The listing builds one solid part. Answer for the finished solid, in the listing's coordinates (mm). Give positions to 0.01 mm unless a question says otherwise; leave off trailing zeros. Write each loop counter-clockwise with the first axis right and the second up, starting at its lowest first coordinate (ties: lowest second). Pieces come first, ordered by that corner, then holes. Notation, with made-up numbers: (-18, 21.5) -> (30, 21.5) arc R14 ccw to (30, 27.5) -> close; hole circle Ø3 at (-34, 84). An arc over 180 degrees is marked (long way). Put each result on its own line as item: value. Start each with the question number.
1) Find the intervals of material crossed by line 1 along X through (y, z) = (2, 1.1); line 2 along Y through (x, z) = (15, -0.6); line 3 along X through (y, z) = (8.5, 0.95), in increasing order. Write a range as from..to.
2) A cutting plane is placed at A-A (y = 15.5). Write down the section's boundary in (x, z), then the cut area to 3 significant figures.
3) A cutting plane is placed at C-C (x = -26.5). Write down the section's boundary in (y, z).
4) A cutting plane is placed at B-B (x = -45.5). Write down the section's boundary in (y, z).
5) Flat-ended cylindrical pins translate along their axes: pin 1 Ø0.9 at (y, z) = (6.5, -1) entering from +X; pin 2 Ø0.5 at (y, z) = (4.5, -0.5) entering from +X; pin 3 Ø3 at (x, y) = (-41.61, 16.5) entering from -Z; pin 4 Ø1.1 at (x, z) = (-32, 0.5) entering from -Y. Find the tip coordinate at first contact, or state that the pin passes through.
Autodesk Inventor part; units mm, degrees
sketch "Эскиз1" plane through (0, 0, 0) normal (0, 0, 1) x (1, 0, 0)
  line L0 (-70.2411, 0) -> (14.7589, 0)
  line L1 (14.7589, 0) -> (14.7589, 30)
  line L2 (14.7589, 30) -> (-70.2411, 20)
  line L3 (0, 36) -> (0, -6) construction
  line L4 (-70.2411, 20) -> (-70.2411, 0)
  point P0 (0, 0)
  dimension "d0" = 30
  dimension "d1" = 85
  dimension "d46" = 14.7589
  dimension "d47" = 20
extrude "Выдавливание1" add sketch "Эскиз1" along normal mid plane 4
sketch "Эскиз2" plane through (-70.2411, 0, 2) normal (0, -1, 0) x (1, 0, 0)
  line L0 (0, -4) -> (0, 0)
  line L1 (85, 0) -> (0, 0)
  line L2 (0, -4) -> (5, -4)
  line L3 (5, -4) -> (5, 0)
  line L4 (5, 0) -> (0, 0)
  line L5 (0, 0) -> (0, -4)
  line L6 (0, -4) -> (85, -4)
  line L7 (15, -4) -> (20, -4)
  line L8 (20, -4) -> (20, 0)
  line L9 (20, 0) -> (15, 0)
  line L10 (15, 0) -> (15, -4)
  line L11 (30, -4) -> (35, -4)
  line L12 (35, -4) -> (35, 0)
  line L13 (35, 0) -> (30, 0)
  line L14 (30, 0) -> (30, -4)
  line L15 (45, -4) -> (50, -4)
  line L16 (50, -4) -> (50, 0)
  line L17 (50, 0) -> (45, 0)
  line L18 (45, 0) -> (45, -4)
  line L19 (85, -4) -> (80, -4)
  line L20 (80, -4) -> (80, 0)
  line L21 (80, 0) -> (85, 0)
  line L22 (85, 0) -> (85, -4)
  line L23 (74, -4) -> (69, -4)
  line L24 (69, -4) -> (69, 0)
  line L25 (69, 0) -> (74, 0)
  line L26 (74, 0) -> (74, -4)
  point P0 (70.2411, -2)
  point P1 (15, 0)
  point P2 (45, 0)
  point P3 (74, 0)
  dimension "d4" = 5
  dimension "d5" = 5
  dimension "d6" = 10
  dimension "d9" = 30
  dimension "d14" = 5
  dimension "d15" = 5
  dimension "d16" = 6
extrude "Выдавливание2" add sketch "Эскиз2" along normal blind 3 contours L0 L1 L3 L2 | L10 L1 L8 L6 | L14 L1 L12 L6 | L18 L1 L16 L6 | L24 L1 L26 L6 | L20 L1 L22 L6
sketch "Эскиз3" plane through (14.7589, 30, 2) normal (1, 0, 0) x (0, 0, -1)
  line L0 (4, 0) -> (0, 0)
  line L1 (4, 0) -> (0, 0)
  line L2 (0, 0) -> (0, -4)
  line L3 (0, -4) -> (4, -4)
  line L4 (4, -4) -> (4, 0)
  line L5 (4, -9) -> (0, -9)
  line L6 (0, -9) -> (0, -13)
  line L7 (0, -13) -> (4, -13)
  line L8 (4, -13) -> (4, -9)
  line L9 (4, 0) -> (4, -33)
  line L10 (4, -10) -> (4, 0)
  line L11 (0, 0) -> (0, -33)
  line L12 (4, -17) -> (0, -17)
  line L13 (0, -17) -> (0, -21)
  line L14 (0, -21) -> (4, -21)
  line L15 (4, -21) -> (4, -17)
  line L16 (4, -26) -> (0, -26)
  line L17 (0, -26) -> (0, -30)
  line L18 (0, -30) -> (4, -30)
  line L19 (4, -30) -> (4, -26)
  point P0 (2, -30)
  point P1 (4, -30)
  point P2 (4, -16.5)
  point P3 (4, -30)
  point P4 (0, -26)
  point P5 (0, -17)
  dimension "d19" = 4
  dimension "d20" = 4
  dimension "d21" = 5
  dimension "d29" = 4
  dimension "d30" = 5
  dimension "d31" = 4
  dimension "d32" = 4
extrude "Выдавливание3" add sketch "Эскиз3" along normal blind 6 contours L4 L3 L2 L0 | L8 L7 L6 L5 | L12 L9 L14 L11 | L16 L9 L18 L11
sketch "Эскиз4" plane through (0, 0, 2) normal (0, 0, 1) x (1, 0, 0)
  line L0 (-0.1411, 5.05) -> (-0.1411, 7.95)
  line L1 (14.7589, 7.95) -> (14.7589, 5.05)
  line L2 (6.6589, 9.3) -> (4.8589, 9.3)
  line L3 (4.8589, 3.7) -> (6.6589, 3.7)
  line L4 (14.7589, 9) -> (14.7589, 4)
  line L5 (14.7589, 6.5) -> (-0.1411, 6.5) construction
  line L6 (-0.1411, 7.95) -> (4.8589, 7.95)
  line L7 (6.6589, 7.95) -> (14.7589, 7.95)
  line L8 (6.6589, 3.7) -> (6.6589, 5.05)
  line L9 (6.6589, 7.95) -> (6.6589, 9.3)
  line L10 (4.8589, 9.3) -> (4.8589, 7.95)
  line L11 (4.8589, 5.05) -> (4.8589, 3.7)
  line L12 (14.7589, 5.05) -> (6.6589, 5.05)
  line L13 (4.8589, 5.05) -> (-0.1411, 5.05)
  line L14 (-0.1411, 22.05) -> (-0.1411, 24.95)
  line L15 (14.7589, 24.95) -> (14.7589, 22.05)
  line L16 (6.6589, 26.3) -> (4.8589, 26.3)
  line L17 (4.8589, 20.7) -> (6.6589, 20.7)
  line L18 (14.7589, 23.5) -> (-0.1411, 23.5) construction
  line L19 (-0.1411, 24.95) -> (4.8589, 24.95)
  line L20 (6.6589, 24.95) -> (14.7589, 24.95)
  line L21 (6.6589, 20.7) -> (6.6589, 22.05)
  line L22 (6.6589, 24.95) -> (6.6589, 26.3)
  line L23 (4.8589, 26.3) -> (4.8589, 24.95)
  line L24 (4.8589, 22.05) -> (4.8589, 20.7)
  line L25 (14.7589, 22.05) -> (6.6589, 22.05)
  line L26 (4.8589, 22.05) -> (-0.1411, 22.05)
  line L27 (14.7589, 26) -> (14.7589, 21)
  point P0 (0, 0)
  dimension "d33" = 2.9
  dimension "d34" = 1.8
  dimension "d35" = 5.6
  dimension "d37" = 1.35
  dimension "d38" = 5
  dimension "d39" = 8.1
  dimension "d40" = 2.9
  dimension "d41" = 1.8
  dimension "d42" = 5.6
  dimension "d43" = 1.35
  dimension "d44" = 5
  dimension "d45" = 8.1
extrude "Выдавливание4" cut sketch "Эскиз4" against normal up to surface (4 mm away)
sketch "Эскиз5" plane through (0, 0, 2) normal (0, 0, 1) x (1, 0, 0)
  line L0 (-61.6911, 0) -> (-58.7911, 0)
  line L1 (-58.7911, 13.9) -> (-61.6911, 13.9)
  line L2 (-31.6911, 0) -> (-28.7911, 0)
  line L3 (-28.7911, 13.9) -> (-31.6911, 13.9)
  line L4 (-60.2411, 0) -> (-60.2411, 13.9) construction
  line L5 (-30.2411, 13.9) -> (-30.2411, 0) construction
  line L6 (-57.4411, 9.9) -> (-57.4411, 8.1)
  line L7 (-63.0411, 8.1) -> (-63.0411, 9.9)
  line L8 (-27.4411, 9.9) -> (-27.4411, 8.1)
  line L9 (-33.0411, 8.1) -> (-33.0411, 9.9)
  line L10 (-63.0411, 9.9) -> (-61.6911, 9.9)
  line L11 (-58.7911, 9.9) -> (-57.4411, 9.9)
  line L12 (-61.6911, 13.9) -> (-61.6911, 9.9)
  line L13 (-61.6911, 8.1) -> (-61.6911, 0)
  line L14 (-57.4411, 8.1) -> (-58.7911, 8.1)
  line L15 (-61.6911, 8.1) -> (-63.0411, 8.1)
  line L16 (-58.7911, 0) -> (-58.7911, 8.1)
  line L17 (-58.7911, 9.9) -> (-58.7911, 13.9)
  line L18 (-33.0411, 9.9) -> (-31.6911, 9.9)
  line L19 (-28.7911, 9.9) -> (-27.4411, 9.9)
  line L20 (-27.4411, 8.1) -> (-28.7911, 8.1)
  line L21 (-31.6911, 8.1) -> (-33.0411, 8.1)
  line L22 (-31.6911, 13.9) -> (-31.6911, 9.9)
  line L23 (-31.6911, 8.1) -> (-31.6911, 0)
  line L24 (-28.7911, 0) -> (-28.7911, 8.1)
  line L25 (-28.7911, 9.9) -> (-28.7911, 13.9)
  line L26 (-65.2411, 0) -> (-55.2411, 0)
  line L27 (-35.2411, 0) -> (-25.2411, 0)
  point P0 (0, 0)
  dimension "d50" = 1.8
  dimension "d51" = 5.6
  dimension "d52" = 2.9
  dimension "d54" = 1.35
  dimension "d55" = 8.1
  dimension "d56" = 4
extrude "Выдавливание5" cut sketch "Эскиз5" against normal up to surface (4 mm away)
sketch "Эскиз6" plane through (0, 0, -2) normal (0, 0, -1) x (-1, 0, 0)
  circle A0 centre (41.6053, 16.5) radius 2
  point P0 (0, 0)
  dimension "d61" = 4
extrude "Выдавливание6" cut sketch "Эскиз6" against normal up to surface (4 mm away)
properties part number "Ребро жётскости крыла"
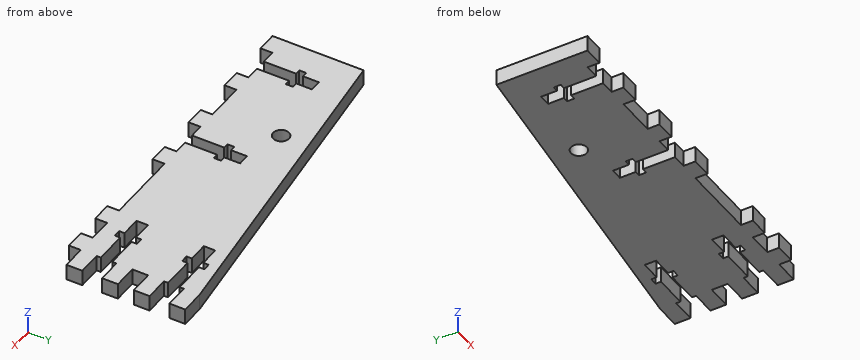
Reply:
1. line 1: x = -70.24..-61.69, -58.79..-31.69, -28.79..20.76
1. line 2: y = 0..4, 9..13, 17..21, 26..30
1. line 3: x = -70.24..-63.04, -57.44..-33.04, -27.44..4.86, 6.66..14.76
2. outline: (-70.24, -2) -> (-43.34, -2) -> (-43.34, 2) -> (-70.24, 2) -> close; (-39.87, -2) -> (14.76, -2) -> (14.76, 2) -> (-39.87, 2) -> close
2. area: 326 mm2
3. outline: (0, -2) -> (25.15, -2) -> (25.15, 2) -> (0, 2) -> close
4. outline: (0, -2) -> (22.91, -2) -> (22.91, 2) -> (0, 2) -> close
5. pin 1: stops at x = -0.14
5. pin 2: stops at x = 14.76
5. pin 3: passes through
5. pin 4: stops at y = 0
